```python
from build123d import *

# Parameters (mm, degrees)
BOSS_EXTRUDE1_DEPTH  = 10
SKETCH2_R            = 1.65
CUT_EXTRUDE1_DEPTH   = 10
FILLET1_R            = 2
FILLET1_OF_MIRROR1_R = 2


with BuildPart() as part:
    # Sketch1 → Boss-Extrude1 (new body)
    with BuildSketch(Plane.XY):
        with BuildLine():
            Line((-21, 0), (-11, 0))
            ThreePointArc((-11, 0), (-7.778174593, 7.778174593), (0, 11))
            Line((0, 11), (0, 16.170747429))
            ThreePointArc((0, 16.170747429), (-10.573391114, 12.235050991), (-16, 2.343730447))
            Line((-16, 2.343730447), (-21, 2.343730447))
            Line((-21, 2.343730447), (-21, 0))
        make_face()
    boss_extrude1 = extrude(amount=BOSS_EXTRUDE1_DEPTH)

    # Sketch2 → Cut-Extrude1 (cut)
    with BuildSketch(Plane(origin=(0, 2.343730447, 0), x_dir=(1, 0, 0), z_dir=(0, 1, 0))):
        with Locations((-18.5, -5)):
            Circle(SKETCH2_R)
    cut_extrude1 = extrude(amount=-CUT_EXTRUDE1_DEPTH, mode=Mode.SUBTRACT)

    # Fillet1
    fillet1_edges = [part.edges().sort_by_distance(p)[0] for p in [
        (-21, 1.171865223, 10),
        (-21, 1.171865223, 0),
    ]]
    fillet(fillet1_edges, radius=FILLET1_R)

    # Mirror1: Boss-Extrude1, Cut-Extrude1 across plane
    add(boss_extrude1.mirror(Plane(origin=(0, 11, 10), x_dir=(0, 0, 1), z_dir=(-1, 0, 0))))
    add(cut_extrude1.mirror(Plane(origin=(0, 11, 10), x_dir=(0, 0, 1), z_dir=(-1, 0, 0))), mode=Mode.SUBTRACT)

    # Fillet1 of Mirror1
    fillet1_of_mirror1_edges = [part.edges().sort_by_distance(p)[0] for p in [
        (21, 1.171865223, 10),
        (21, 1.171865223, 0),
    ]]
    fillet(fillet1_of_mirror1_edges, radius=FILLET1_OF_MIRROR1_R)


solid = part.part
```
Read the model definition and answer for the solid it produces. Units are mm, in the model's axes. A direction names the side the tool comes from. Give positions to 0.01 mm unless a question says otherwise; leave off trailing zeros. Write each loop counter-clockwise with the first axis right and the second up, starting at its lowest first coordinate (ties: lowest second). Pieces come first, ordered by that corner, then holes. Notation, with made-up numbers: (17, 47.25) -> (53, 47.25) arc R11 ccw to (53, 62.25) -> close; hole circle Ø10 at (16.5, -4). An arc over 180 degrees is marked (long way). Answer as a JSON object with one key per item and string values.
1) Section B-B on z = 5 is taken. Write down the section's boundary in (x, y), then the cut area to 3 significant figures.
Findings below:
{"outline": "(-21, 0) -> (-20.15, 0) -> (-20.15, 2.34) -> (-21, 2.34) -> close; (-16.85, 0) -> (-11, 0) arc R11 cw to (11, 0) -> (16.85, 0) -> (16.85, 2.34) -> (16, 2.34) arc R16.17 ccw to (-16, 2.34) -> (-16.85, 2.34) -> close; (20.15, 0) -> (21, 0) -> (21, 2.34) -> (20.15, 2.34) -> close", "area": "228 mm^2"}
2) Section A-A on x = -18.5 is taken. Write down the section's boundary in (y, z).
Findings below:
{"outline": "(0, 0) -> (2.34, 0) -> (2.34, 3.35) -> (0, 3.35) -> close; (0, 6.65) -> (2.34, 6.65) -> (2.34, 10) -> (0, 10) -> close"}
3) Flat-ended cylindrical pins translate along their axes: pin 1 Ø3 at (x, z) = (-18.5, 5) entering from +Y; pin 2 Ø1 at (x, z) = (9.5, 8.5) entering from +Y; pin 3 Ø1 at (y, z) = (5, 4) entering from -X; pin 4 Ø4 at (x, z) = (-19.5, 4.5) entering from +Y. Find the tip coordinate at first contact, or state that the pin passes through.
Findings below:
{"pin 1": "passes through", "pin 2": "stops at y = 13.43", "pin 3": "stops at x = -15.53", "pin 4": "stops at y = 2.34"}
4) A tool of negligible diameter and unlimited length cuts with its end or side. For faces 4 (the flat face through (-17, 2.344, 4)), 5 (the flat face through (17, 2.344, 4)), 6 (the flat face through (-21, 1, 5)), from which of +Z, -Z, +X, -X, +Y, -Y can it reach the whole face along a straight path? Write none if from no direction.
Findings below:
{"face 4": "+Z, -Z, -X, +Y", "face 5": "+Z, -Z, +X, +Y", "face 6": "+Z, -Z, -X, +Y, -Y"}
5) For a pull along Z with two mould halves and no side action, classify faces 1 (the flat face through (0, 12, 0)), 2 (the flat face through (16, 0, 5)), 3 (the cylindrical face through (-19.81, 1.19, 6)) as pulls with the +Z half, pulls with the -Z half, needs draft (parallel to the pull), parting line crosses it, or undercut.
Findings below:
{"face 1": "pulls with the -Z half", "face 2": "needs draft", "face 3": "undercut"}
6) Section C-C on y = 3.5 is taken. Write down the section's boundary in (x, z), then the cut area to 3 significant figures.
Findings below:
{"outline": "(-15.79, 0) -> (-10.43, 0) -> (-10.43, 10) -> (-15.79, 10) -> close; (10.43, 0) -> (15.79, 0) -> (15.79, 10) -> (10.43, 10) -> close", "area": "107 mm^2"}
7) Straight lines are drawn through the part: probe 1 along X at (y, z) = (0.5, 5); probe 2 along X at (y, z) = (1.15, 5); probe 3 along Z at (x, y) = (-18.5, 1.25). For each, find the intervals that lie inside material, in ascending order. Write a range as from..to.
Findings below:
{"probe 1": "x = -21..-20.15, -16.85..-10.99, 10.99..16.85, 20.15..21", "probe 2": "x = -21..-20.15, -16.85..-10.94, 10.94..16.85, 20.15..21", "probe 3": "z = 0..3.35, 6.65..10"}
8) Section D-D on x = -11.5 is taken. Write down the section's boundary in (y, z), then the cut area to 3 significant figures.
Findings below:
{"outline": "(0, 0) -> (11.37, 0) -> (11.37, 10) -> (0, 10) -> close", "area": "114 mm^2"}
